from build123d import *

# Parameters (mm, degrees)
REVOLVE2_ANGLE          = 180
CUT_EXTRUDE1_DEPTH      = 6.477
CUT_EXTRUDE1_DEPTH_BACK = 6.477


# Read off the part's stored shape, not the designer's step: Revolve2
with BuildPart() as part:
    # Revolve2 outline → Revolve2 (revolve)
    with BuildSketch(Plane.XZ):
        Polygon((3.81, 0), (0, 0), (0, -3.81), (38.1, -41.91), (41.91, -41.91), (41.91, -38.1), align=None)
    revolve(axis=Axis((0, 0, 0), (0, 0, 1)), revolution_arc=REVOLVE2_ANGLE)

    # Sketch6 → Cut-Extrude1 (cut, two sides: drawn at the far end of the back side and taken through both)
    with BuildSketch(Plane(origin=(0, 0, 0), x_dir=(0, 0, -1), z_dir=(1, 0, 0)).offset(-CUT_EXTRUDE1_DEPTH_BACK)):
        Polygon((20.066, 20.066), (20.066, 29.318948776), (20.066, 36.223650293), (30.48, 36.223650293), (30.48, 30.48), align=None)
    extrude(amount=CUT_EXTRUDE1_DEPTH + CUT_EXTRUDE1_DEPTH_BACK, mode=Mode.SUBTRACT)


solid = part.part
Check sheet for the modelled part. Datum: model origin and axes. Units: mm. A direction names the side the tool comes from. Give positions to 0.01 mm unless a question says otherwise; leave off trailing zeros. Loops run counter-clockwise (first coordinate to the right, second up) from the corner with the lowest first, then second, coordinate; pieces in that order, holes last. Notation, with made-up numbers: M 41,58 L 53,58 A11 cw 53,70 Z; hole C -10,69.25 d6. An arc over 180 degrees is marked long. Return JSON: item names as keys, results as strings. Group by question number.
1. Cross-section at D-D on z = -7. Record the boundary of the cut face in (x, y).
2. Cross-section at C-C on z = -34. Record the boundary of the cut face in (x, y), plus the area to 3 significant figures.
3. Cross-section at A-A on x = 0. Record the boundary of the cut face in (y, z), plus the area to 3 significant figures.
4. Mould release check, pull along X, two halves, no side actions. Record for faces 3 (the flat face through (0, 2, 0)), 4 (the flat face through (-6.477, 27, -25)), 5 (the conical face through (0.404, 18.356, -14.55)), 6 (the flat face through (0, 32, -30.48)): released by +X, released by -X, zero draft, split by the parting line, or undercut.
5. Go/stop test with flat-tipped pins: pin 1 (3 mm diameter, centred on x = 6, z = -23, fed in from +Y); pin 2 (1.1 mm diameter, centred on x = 1.5, y = 22.5, fed in from -Z); pin 3 (3 mm diameter, centred on x = 11, y = 34, fed in from +Z); pin 4 (3 mm diameter, centred on y = 29.5, z = -23.5, fed in from -X). Record where each tip stops, or that it passes through.
6. Tool access check on faces 1 (the conical face through (0.332, 15.08, -18.893)), 2 (the flat face through (0, 25, -25)). Record the directions out of +Z, -Z, +X, -X, +Y, -Y that give a thin tool (end or side, any length) a straight path to the whole face; none if there is none.
7. Thickness scan on L1, parallel to X at y = 17.5, z = -27; L2, parallel to X at y = 4, z = -24; L3, parallel to Z at x = -25.5, y = 4.5. Record the ranges inside material, lowest first.
8. Cross-section at B-B on z = -25. Record the boundary of the cut face in (x, y), plus the area to 3 significant figures.
Return value:
{
 "1": {"outline": "M -10.81,0 L -3.19,0 A3.19 cw 3.19,0 L 10.81,0 A10.81 ccw Z"},
 "2": {"outline": "M -37.81,0 L -30.19,0 A30.19 cw 30.19,0 L 37.81,0 A37.81 ccw Z", "area": "814 mm^2"},
 "3": {"outline": "M 0,-3.81 L 38.1,-41.91 L 41.91,-41.91 L 41.91,-38.1 L 34.29,-30.48 L 30.48,-30.48 L 20.07,-20.07 L 23.88,-20.07 L 3.81,0 L 0,0 Z", "area": "265 mm^2"},
 "4": {"face 3": "zero draft", "face 4": "undercut", "face 5": "split by the parting line", "face 6": "undercut"},
 "5": {"pin 1": "y = 27.48", "pin 2": "z = -26.91", "pin 3": "z = -30.43", "pin 4": "through"},
 "6": {"face 1": "-Z, -Y", "face 2": "+Y"},
 "7": {"L1": "-25.36 to -15.22, 15.22 to 25.36", "L2": "-27.52 to -19.79, 19.79 to 27.52", "L3": "-29.7 to -22.08"},
 "8": {"outline": "M -28.81,0 L -21.19,0 A21.19 cw 21.19,0 L 28.81,0 A28.81 ccw 6.48,28.07 L 6.48,25 L -6.48,25 L -6.48,28.07 A28.81 ccw Z", "area": "552 mm^2"}
}
